Work out the finished part from the listing and answer in its coordinate system (mm). Face numbers are marked on the shaded views. A direction names the side the tool comes from. Coordinates: 2 decimals unless noted, no trailing zeros. Loops run counter-clockwise (first coordinate to the right, second up) from the corner with the lowest first, then second, coordinate; pieces in that order, holes last.
```python
from build123d import *

# Parameters (mm, degrees)
SKETCH1_W           = 50.8
SKETCH1_H           = 66.96
BOSS_EXTRUDE1_DEPTH = 7
SKETCH2_W           = 20
SKETCH2_H           = 40
CUT_EXTRUDE1_DEPTH  = 7
SKETCH3_W           = 50.8
SKETCH3_H           = 7
BOSS_EXTRUDE2_DEPTH = 69.2
FILLET2_RADIUS      = 25.4
FILLET2_LENGTH      = 7
FILLET3_RADIUS      = 25.4
FILLET3_LENGTH      = 7
SKETCH4_R           = 5
CUT_EXTRUDE2_DEPTH  = 400
FILLET5_R           = 2.54


with BuildPart() as part:
    # Sketch1 → Boss-Extrude1 (new body)
    with BuildSketch(Plane(origin=(0, 0, 0), x_dir=(1, 0, 0), z_dir=(0, 1, 0))):
        Rectangle(SKETCH1_W, SKETCH1_H)
    extrude(amount=BOSS_EXTRUDE1_DEPTH)

    # Sketch2 → Cut-Extrude1 (cut)
    with BuildSketch(Plane(origin=(0, 7, 0), x_dir=(1, 0, 0), z_dir=(0, 1, 0))):
        Rectangle(SKETCH2_W, SKETCH2_H)
    extrude(amount=-CUT_EXTRUDE1_DEPTH, mode=Mode.SUBTRACT)

    # Sketch3 → Boss-Extrude2 (add)
    with BuildSketch(Plane(origin=(0, 7, 0), x_dir=(1, 0, 0), z_dir=(0, 1, 0))):
        with Locations((0, 29.98)):
            Rectangle(SKETCH3_W, SKETCH3_H)
        with Locations((0, -29.98)):
            Rectangle(SKETCH3_W, SKETCH3_H)
    extrude(amount=BOSS_EXTRUDE2_DEPTH)

    # Fillet2: full round fillet: the end face becomes a half cylinder, R = half its width
    fillet2_face = Plane((0, 76.2, -29.98), x_dir=(0, 0, 1), z_dir=(0, 1, 0))  # on the end face: x along it, z out of the body
    fillet2_slab = fillet2_face.offset(-FILLET2_RADIUS / 2) * Box(FILLET2_LENGTH, 2 * FILLET2_RADIUS, FILLET2_RADIUS, mode=Mode.PRIVATE)  # the body's end, R deep
    fillet2_round = Plane((0, 50.8, -29.98), x_dir=(0, 1, 0), z_dir=(0, 0, 1)) * Cylinder(FILLET2_RADIUS, FILLET2_LENGTH, mode=Mode.PRIVATE)  # its axis R under the face
    add(fillet2_slab - fillet2_round, mode=Mode.SUBTRACT)

    # Fillet3: full round fillet: the end face becomes a half cylinder, R = half its width
    fillet3_face = Plane((0, 76.2, 29.98), x_dir=(0, 0, -1), z_dir=(0, 1, 0))  # on the end face: x along it, z out of the body
    fillet3_slab = fillet3_face.offset(-FILLET3_RADIUS / 2) * Box(FILLET3_LENGTH, 2 * FILLET3_RADIUS, FILLET3_RADIUS, mode=Mode.PRIVATE)  # the body's end, R deep
    fillet3_round = Plane((0, 50.8, 29.98), x_dir=(0, 1, 0), z_dir=(0, 0, -1)) * Cylinder(FILLET3_RADIUS, FILLET3_LENGTH, mode=Mode.PRIVATE)  # its axis R under the face
    add(fillet3_slab - fillet3_round, mode=Mode.SUBTRACT)

    # Sketch4 → Cut-Extrude2 (cut, symmetric)
    with BuildSketch(Plane.XY.offset(-26.48)):
        with Locations((0, 50.8)):
            Circle(SKETCH4_R)
    extrude(amount=CUT_EXTRUDE2_DEPTH, both=True, mode=Mode.SUBTRACT)

    # Fillet5
    fillet5_edges = [part.edges().sort_by_distance(p)[0] for p in [
        (0, 7, -26.48),
        (0, 7, 26.48),
        (0, 0, -33.48),
        (0, 0, 33.48),
    ]]
    fillet(fillet5_edges, radius=FILLET5_R)


solid = part.part
```
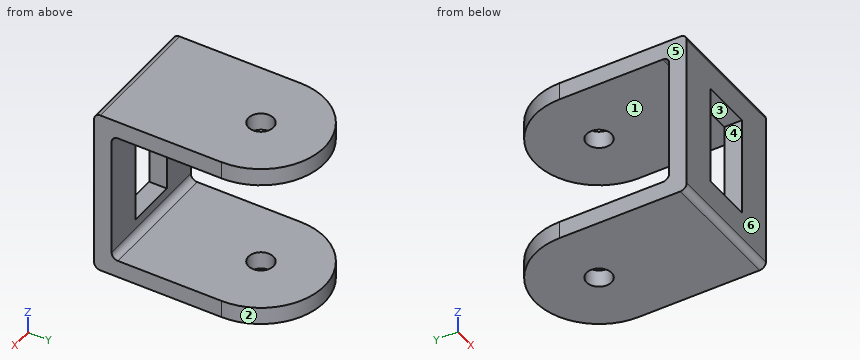
1. Determine the mould class of the marked faces 4, 5 and 6 for opening direction X: released by +X, released by -X, zero draft, split by the parting line, or undercut.
2. Straight lines are drawn through the part: probe 1 along Z at (x, y) = (19, 36); probe 2 along Y at (x, z) = (0, 29.25); probe 3 along Y at (x, z) = (14, 24). For each, find the intervals that lie inside material, in ascending order.
3. A cutting plane is placed at B-B, the plane z = 2. Give the vertices of the cut face in (x, y).
4. For the marked faces 1, 2 and 3, determine the directions among +Z, -Z, +X, -X, +Y, -Y from which every point of the face is accessible in a straight line to the end or side of a thin tool.
5. Each of these flat-tipped pins is pushed along its axis until it touches: P1, Ø11.5, axis at x = 0, y = 50.8, coming from the +Z side; P2, Ø24, axis at x = -9.5, z = -8.5, coming from the +Y side; P3, Ø4, axis at x = -15, z = -23.5, coming from the +Y side. Where does it stop, or does it pass through?
6. A cutting plane is placed at A-A, the plane x = 0. Give the vertices of the cut face in (y, z).
7. A cutting plane is placed at C-C, the plane y = 24.5. Give the vertices of the cut face in (x, z).
8. A cutting plane is placed at D-D, the plane z = 28. Give the vertices of the cut face in (x, y), then the cut area to 3 significant figures.
Answers below:
1. face 4: undercut
1. face 5: released by -X
1. face 6: zero draft
2. probe 1: z = -33.48 to -26.48, 26.48 to 33.48
2. probe 2: y = 0 to 45.8, 55.8 to 76.2
2. probe 3: y = 0 to 7
3. outline: (-25.4, 0) - (-10, 0) - (-10, 7) - (-25.4, 7) - close; (10, 0) - (25.4, 0) - (25.4, 7) - (10, 7) - close
4. face 1: +X, -X, +Y
4. face 2: +Z, -Z, +Y
4. face 3: +Y, -Y
5. P1: stops at z = 33.48
5. P2: stops at y = 7
5. P3: stops at y = 7.54
6. outline: (0, -30.94) arc R2.54 ccw to (2.54, -33.48) - (45.8, -33.48) - (45.8, -26.48) - (9.54, -26.48) arc R2.54 cw to (7, -23.94) - (7, -20) - (0, -20) - close; (0, 20) - (7, 20) - (7, 23.94) arc R2.54 cw to (9.54, 26.48) - (45.8, 26.48) - (45.8, 33.48) - (2.54, 33.48) arc R2.54 ccw to (0, 30.94) - close; (55.8, -33.48) - (76.2, -33.48) - (76.2, -26.48) - (55.8, -26.48) - close; (55.8, 26.48) - (76.2, 26.48) - (76.2, 33.48) - (55.8, 33.48) - close
7. outline: (-25.4, -33.48) - (25.4, -33.48) - (25.4, -26.48) - (-25.4, -26.48) - close; (-25.4, 26.48) - (25.4, 26.48) - (25.4, 33.48) - (-25.4, 33.48) - close
8. outline: (-25.4, 0) - (25.4, 0) - (25.4, 50.8) arc R25.4 ccw to (-25.4, 50.8) - close; hole circle Ø10 at (0, 50.8)
8. area: 3,520 mm2
